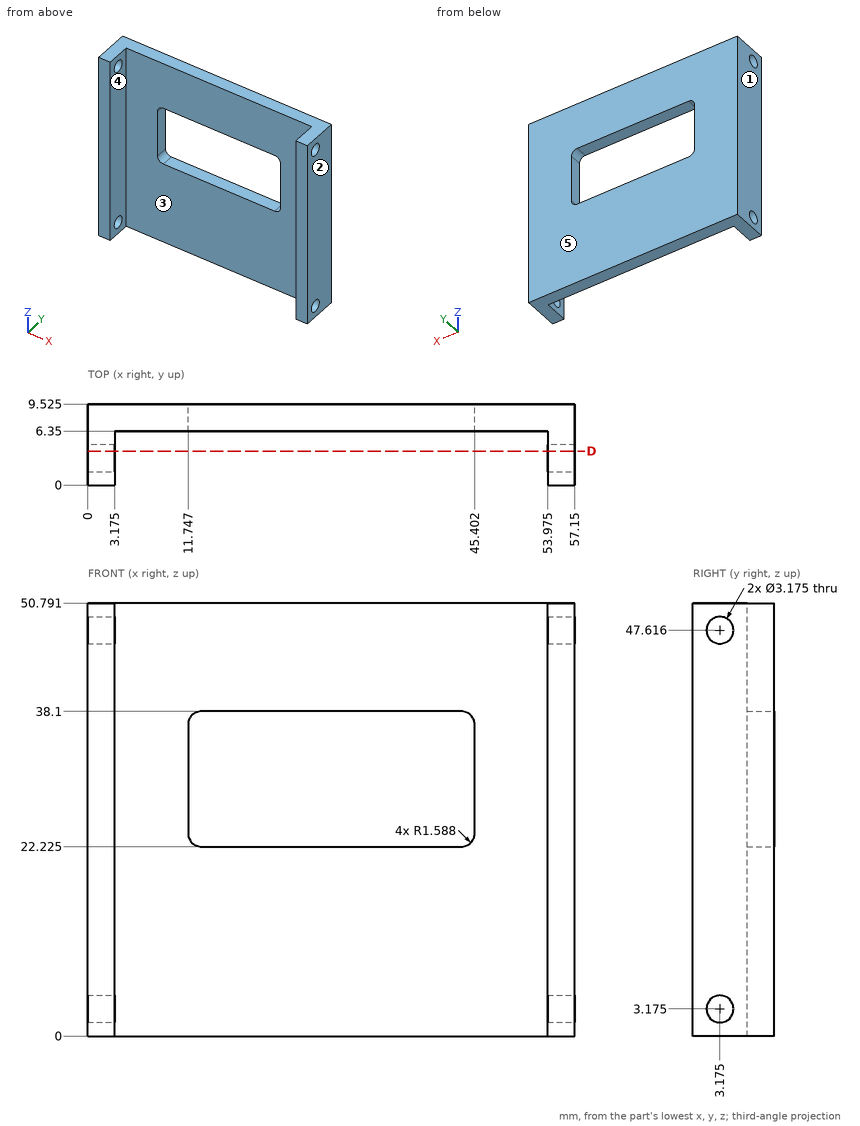
Input: dimensioned drawing with shaded views. Units: mm. Origin: part minimum x, y, z. A direction names the side the tool comes from. Coordinates: 2 decimals unless noted, no trailing zeros. Use a Markdown table: item, result. Add a question column.
(1) Line query: line 1 along Z through (x, y) = (40, 7.25) (1 decimal); line 2 along X through (y, z) = (7.5, 36); line 3 along X through (y, z) = (7, 23). Output: solid intervals per line, ascending.
(2) Pin query (flat end, axial travel): pin 1 Ø12 at (x, z) = (38, 22.5) entering from -Y; pin 2 Ø1.9 at (y, z) = (3.175, 3.175) entering from -X. Return the tip coordinate at first contact, or that it passes through.
(3) Section query D-D, the plane y = 4. State how many separate pieces and enclosed holes the cut face has, plus the area to 3 significant figures.
(4) Mould query, pull axis X, two halves, no side actions, for the marked faces 1, 2 and 3. Classes: pulls with the +X half, pulls with the -X half, needs draft (parallel to the pull), parting line crosses it, or undercut.
(5) Access query for the marked faces 4 and 5. Directions: +Z, -Z, +X, -X, +Y, -Y. A direction counts if a zero-diameter tool reaches every point of the face in a straight line with its end or side. Return the directions, or none.
Answer:
| question | item | result |
|---|---|---|
| 1 | line 1 | z = 0 to 22.2, 38.1 to 50.8 |
| 1 | line 2 | x = 0 to 11.75, 45.4 to 57.15 |
| 1 | line 3 | x = 0 to 11.97, 45.18 to 57.15 |
| 2 | pin 1 | stops at y = 6.35 |
| 2 | pin 2 | passes through |
| 3 | separate pieces | 6 |
| 3 | enclosed holes | 0 |
| 3 | area | 288 mm^2 |
| 4 | face 1 | pulls with the -X half |
| 4 | face 2 | pulls with the +X half |
| 4 | face 3 | undercut |
| 5 | face 4 | +Z, -Z, -Y |
| 5 | face 5 | +Z, -Z, +X, -X, +Y |
